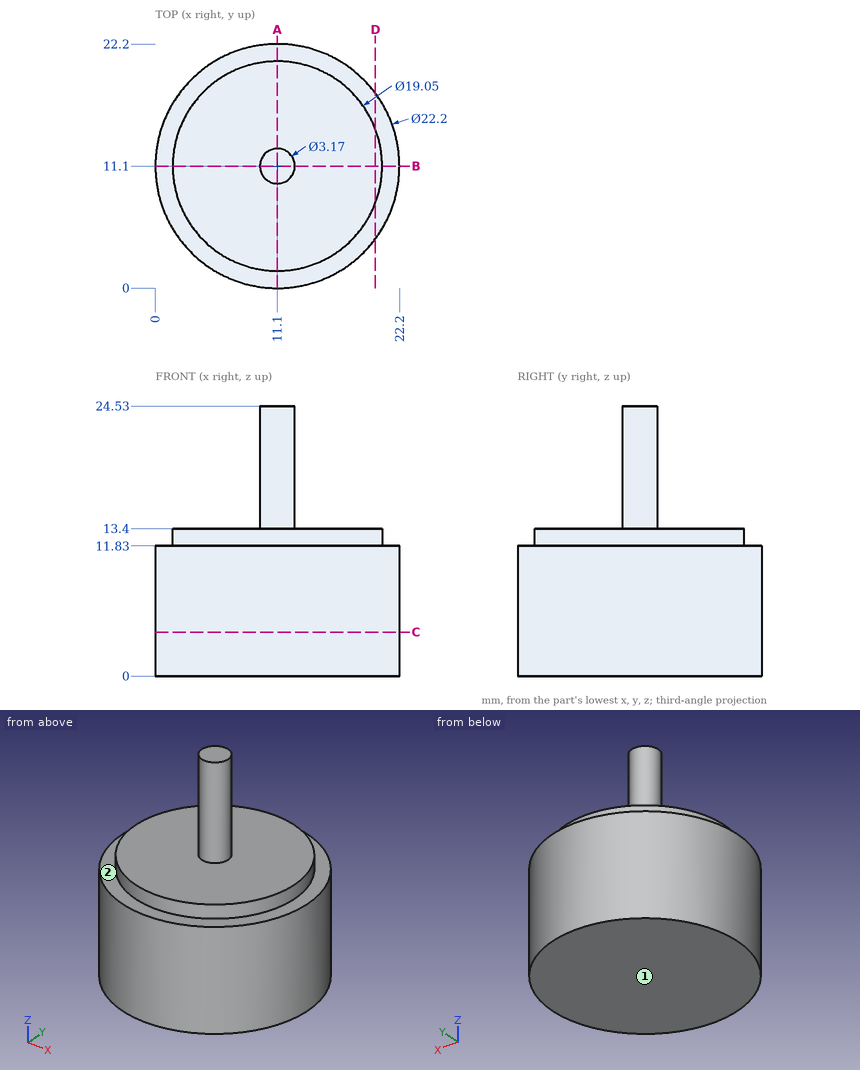
Drawing for the job (mm, zero at the part's lowest x, y, z). A direction names the side the tool comes from. Give positions to 0.01 mm unless a question says otherwise; leave off trailing zeros. Order: outer loops, then holes, each group sorted by start corner. A loop starts at its lowest first (then second) coordinate and runs counter-clockwise, first axis right, second up. Notation, with made-up numbers: (20, -36) - (42, -36) arc R16 cw to (42, -11) - close; hole circle Ø10 at (52, 32). An arc over 180 degrees is marked (long way). Write item = value, one per line. Start each with the question number.
1. Drop flat-ended pins along their axis: P1, Ø2, axis at x = 3, y = 17.5, coming from the +Z side; P2, Ø6, axis at x = 9.5, z = 20.5, coming from the +Y side (3 decimals); P3, Ø1.5, axis at y = 8.5, z = 11, coming from the -X side. Give the stop position or say it passes through.
2. Cut at D-D, the plane x = 20. List the corners of the cut face in (y, z), and give its area (3 significant figures).
3. Which spindle directions (+Z, -Z, +X, -X, +Y, -Y) get a long thin tool onto all of the face, cutting with end or side? Do the marked faces 1 and 2. Say none if no direction does.
4. Probe line 1 along Z through (x, y) = (12.5, 15.25); line 2 along Z through (x, y) = (16.5, 1.5); line 3 along Y through (x, z) = (11.25, 20). List the from-to ranges inside material, lowest first.
5. Cut at A-A, the plane x = 11.1. List the corners of the cut face in (y, z) (3 decimals), and give its area (3 significant figures).
6. Cut at C-C, the plane z = 4. List the corners of the cut face in (x, y).
Taken from the geometry:
q1.P1 = 13.4
q1.P2 = 12.685
q1.P3 = 0.16
q2.outline = (4.47, 0) - (17.73, 0) - (17.73, 11.83) - (14.49, 11.83) - (14.49, 13.4) - (7.71, 13.4) - (7.71, 11.83) - (4.47, 11.83) - close
q2.area = 168 mm²
q3.face_1 = -Z, +X, -X, +Y, -Y
q3.face_2 = +Z
q4.line_1 = 0 to 13.4
q4.line_2 = 0 to 11.83
q4.line_3 = 9.52 to 12.68
q5.outline = (0, 0) - (22.2, 0) - (22.2, 11.83) - (20.625, 11.83) - (20.625, 13.4) - (12.685, 13.4) - (12.685, 24.53) - (9.515, 24.53) - (9.515, 13.4) - (1.575, 13.4) - (1.575, 11.83) - (0, 11.83) - close
q5.area = 328 mm²
q6.outline = circle Ø22.2 at (11.1, 11.1)
